Job drawing, mm, ordinate dimensions from the low corner. One solid piece. Give positions to 0.01 mm unless a question says otherwise; leave off trailing zeros. Order: outer loops, then holes, each group sorted by start corner. A loop starts at its lowest first (then second) coordinate and runs counter-clockwise, first axis right, second up. Notation, with made-up numbers: M -29.5,-1.75 L 23.5,-1.75 A25 cw 23.5,34.25 Z; hole C 23.25,41.25 d10. An arc over 180 degrees is marked long. One line per question, with ' | ' between items.
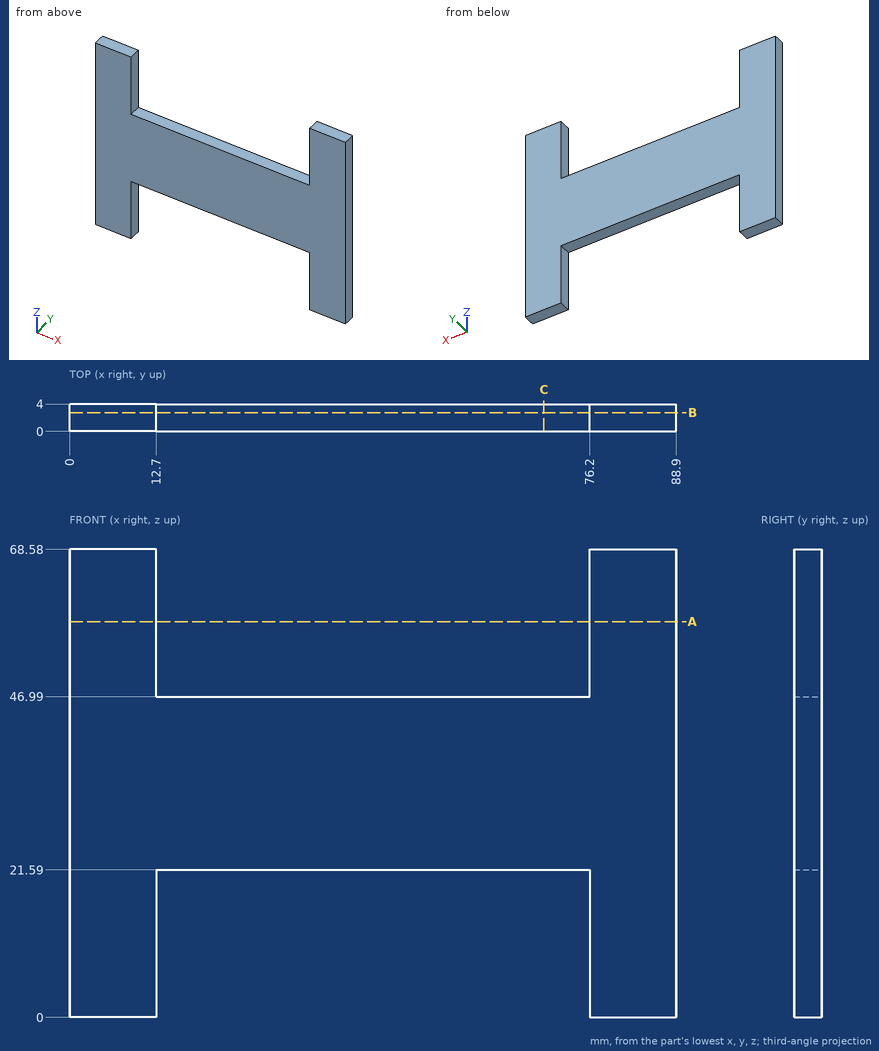
1. Slice it at C-C on x = 69.5. Give the cut face in (y, z).
Worked out:
outline: M 0,21.59 L 4,21.59 L 4,46.99 L 0,46.99 Z
2. Slice it at A-A on z = 58. Give the cut face in (x, y).
Worked out:
outline: M 0,0 L 12.7,0 L 12.7,4 L 0,4 Z; M 76.2,0 L 88.9,0 L 88.9,4 L 76.2,4 Z
3. Probe L1, parallel to X at y = 3.75, z = 14.5; L2, parallel to Z at x = 42.5, y = 2.85. List the from-to ranges inside material, lowest first. Write a range as from..to.
Worked out:
L1: x = 0..12.7, 76.2..88.9 | L2: z = 21.59..46.99
4. Slice it at B-B on y = 2.75. Give the cut face in (x, z), then the cut area to 3 significant figures.
Worked out:
outline: M 0,0 L 12.7,0 L 12.7,21.59 L 76.2,21.59 L 76.2,0 L 88.9,0 L 88.9,68.58 L 76.2,68.58 L 76.2,46.99 L 12.7,46.99 L 12.7,68.58 L 0,68.58 Z | area: 3,350 mm2
5. Drop flat-ended pins along their axis: pin 1 (2 mm diameter, centred on x = 66.5, y = 0.5, fed in from +Z); pin 2 (2 mm diameter, centred on x = 76.5, z = 60.5, fed in from -Y). Give the stop position or say it passes through.
Worked out:
pin 1: stops at z = 46.99 | pin 2: stops at y = 0
